For this review, take the finished solid that the model builds, in its own axes (mm). A direction names the side the tool comes from. Give positions to 0.01 mm unless a question says otherwise; leave off trailing zeros. Write each loop counter-clockwise with the first axis right and the second up, starting at its lowest first coordinate (ties: lowest second). Pieces come first, ordered by that corner, then holes. Notation, with made-up numbers: (-36, 60.5) -> (-8, 60.5) arc R16 ccw to (-8, 80.5) -> close; hole circle Ø10 at (-8.5, -13.75). An arc over 180 degrees is marked (long way). Return JSON: item names as keys, results as strings.
from build123d import *

# Parameters (mm, degrees)
F0_W     = 7.62
F0_H     = 24.13
F0_R     = 2.159
F0_R_2   = 1.8
F2_DEPTH = 12.7
F1_W     = 0.635
F1_H     = 15.24
F3_DEPTH = 19.05
F4_SIZE  = 0.635
F5_W     = 19.05
F5_H     = 5.08
F6_DEPTH = 12.7


with BuildPart() as f2:
    # F0 (on Top) → F2 (new body)
    with BuildSketch(Plane.XY):
        with Locations((0, -12.065)):
            Rectangle(F0_W, F0_H)
        with Locations((0, -15.24)):
            Circle(F0_R, mode=Mode.SUBTRACT)
        with Locations((0, -2.794)):
            Circle(F0_R_2, mode=Mode.SUBTRACT)
    extrude(amount=F2_DEPTH)

    # F1 (on Top) → F3 (cut)
    with BuildSketch(Plane.XY):
        with Locations((0, -7.62)):
            Rectangle(F1_W, F1_H)
    extrude(amount=F3_DEPTH, mode=Mode.SUBTRACT)

    # F4
    f4_edges = [f2.edges().sort_by_distance(p)[0] for p in [
        (0.3175, 0, 6.35),
        (-0.3175, 0, 6.35),
    ]]
    chamfer(f4_edges, length=F4_SIZE)

    # F5 (on Right) → F6 (cut, symmetric)
    with BuildSketch(Plane.YZ):
        with Locations((-9.525, 2.54)):
            Rectangle(F5_W, F5_H)
    extrude(amount=F6_DEPTH, both=True, mode=Mode.SUBTRACT)


solid = f2.part
1. Add section A-A, the plane y = -9.25. State the section outline as (x, z) points, plus the area to 3 significant figures.
Results found:
{"outline": "(-3.81, 5.08) -> (-0.32, 5.08) -> (-0.32, 12.7) -> (-3.81, 12.7) -> close; (0.32, 5.08) -> (3.81, 5.08) -> (3.81, 12.7) -> (0.32, 12.7) -> close", "area": "53.2 mm²"}
2. For faces 1 (the flat face through (-0.318, -9, 9)), 2 (the cylindrical face through (-1.8, -2.8, 8.8)), 3 (the flat face through (2, 0, 9)), 4 (the flat face through (-3.81, -15, 8)), 5 (the flat face through (0, -19.05, 3)), list the 3-axis set-ups (+Z, -Z, +X, -X, +Y, -Y) from which the entire face can be reached by the end or side of a thin tool; tool diameter is ignored.
Results found:
{"face 1": "+Z, -Z, +Y", "face 2": "+Z, -Z", "face 3": "+Z, -Z, +X, -X, +Y", "face 4": "+Z, -Z, -X, +Y, -Y", "face 5": "-Z, +X, -X, +Y"}
3. To check wall thickness, follow probe 1 along X at (y, z) = (-15.24, 9.25); probe 2 along X at (y, z) = (-5.25, 7.5); probe 3 along Z at (x, y) = (2.5, -14). State the ranges of each line that lie inside material, in increasing order.
Results found:
{"probe 1": "x = -3.81 to -2.16, 2.16 to 3.81", "probe 2": "x = -3.81 to -0.32, 0.32 to 3.81", "probe 3": "z = 5.08 to 12.7"}
4. Add section D-D, the plane x = 1.5. State the section outline as (y, z) points, plus the area to 3 significant figures.
Results found:
{"outline": "(-24.13, 0) -> (-19.05, 0) -> (-19.05, 5.08) -> (-16.79, 5.08) -> (-16.79, 12.7) -> (-24.13, 12.7) -> close; (-13.69, 5.08) -> (-3.79, 5.08) -> (-3.79, 12.7) -> (-13.69, 12.7) -> close; (-1.8, 5.08) -> (0, 5.08) -> (0, 12.7) -> (-1.8, 12.7) -> close", "area": "171 mm²"}
5. For pin 1 (4 mm diameter, centred on x = -0.5, z = 1.5, fed in from +Y), flat-tipped, find the tip position at first contact; note if it passes through.
Results found:
{"pin 1": "stops at y = -19.05"}
6. Add section C-C, the plane y = -15.24. State the section outline as (x, z) points, plus the area to 3 significant figures.
Results found:
{"outline": "(-3.81, 5.08) -> (-2.16, 5.08) -> (-2.16, 12.7) -> (-3.81, 12.7) -> close; (2.16, 5.08) -> (3.81, 5.08) -> (3.81, 12.7) -> (2.16, 12.7) -> close", "area": "25.2 mm²"}
